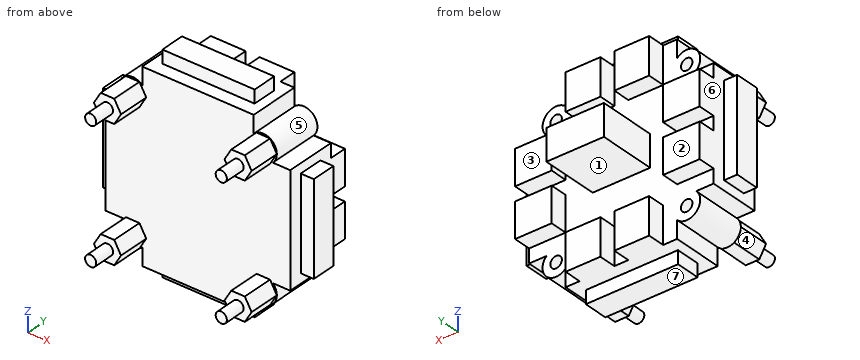
from build123d import *

# Parameters (mm, degrees)
SKETCH_1_R        = 3.889087297
SKETCH_1_R_2      = 1.65
EXTRUDE_2_DEPTH   = 7.25
EXTRUDE_2_2_DEPTH = 7.25
EXTRUDE_2_3_DEPTH = 7.25
EXTRUDE_2_4_DEPTH = 7.25
SKETCH_2_W        = 32
SKETCH_2_H        = 53
SKETCH_2_W_2      = 53
SKETCH_2_H_2      = 32
EXTRUDE_3_DEPTH   = 7.25
SKETCH_3_W        = 26.5
SKETCH_3_H        = 60.5
SKETCH_3_W_2      = 60.5
SKETCH_3_H_2      = 26.5
EXTRUDE_4_DEPTH   = 3.5
SKETCH_4_W        = 16.5
SKETCH_4_H        = 9
EXTRUDE_5_DEPTH   = 16.5
SKETCH_5_W        = 10.5
SKETCH_5_H        = 10
SKETCH_5_W_2      = 10
SKETCH_5_H_2      = 10.5
EXTRUDE_6_DEPTH   = 5
EXTRUDE_7_DEPTH   = 9
SKETCH_7_R        = 1.6
EXTRUDE_8_DEPTH   = 6


with BuildPart() as part:
    # Sketch 1 → Extrude 2 (new, symmetric)
    with BuildSketch(Plane(origin=(0, 0, 0), x_dir=(1, 0, 0), z_dir=(0, 1, 0))):
        with Locations(Location((-18.75, 18.75, 0), (0, 0, 90))):
            Circle(SKETCH_1_R)
        with Locations(Location((-18.75, 18.75, 0), (0, 0, 90))):
            Circle(SKETCH_1_R_2, mode=Mode.SUBTRACT)
    extrude(amount=EXTRUDE_2_DEPTH, both=True)



with BuildPart() as body_2:
    # Sketch 1 → Extrude 2 2 (new, symmetric)
    with BuildSketch(Plane(origin=(0, 0, 0), x_dir=(1, 0, 0), z_dir=(0, 1, 0))):
        with Locations(Location((18.75, 18.75, 0), (0, 0, 90))):
            Circle(SKETCH_1_R)
        with Locations(Location((18.75, 18.75, 0), (0, 0, 90))):
            Circle(SKETCH_1_R_2, mode=Mode.SUBTRACT)
    extrude(amount=EXTRUDE_2_2_DEPTH, both=True)


with BuildPart() as body_3:
    # Sketch 1 → Extrude 2 3 (new, symmetric)
    with BuildSketch(Plane(origin=(0, 0, 0), x_dir=(1, 0, 0), z_dir=(0, 1, 0))):
        with Locations(Location((18.75, -18.75, 0), (0, 0, 90))):
            Circle(SKETCH_1_R)
        with Locations(Location((18.75, -18.75, 0), (0, 0, 90))):
            Circle(SKETCH_1_R_2, mode=Mode.SUBTRACT)
    extrude(amount=EXTRUDE_2_3_DEPTH, both=True)


with BuildPart() as body_4:
    # Sketch 1 → Extrude 2 4 (new, symmetric)
    with BuildSketch(Plane(origin=(0, 0, 0), x_dir=(1, 0, 0), z_dir=(0, 1, 0))):
        with Locations(Location((-18.75, -18.75, 0), (0, 0, 90))):
            Circle(SKETCH_1_R)
        with Locations(Location((-18.75, -18.75, 0), (0, 0, 90))):
            Circle(SKETCH_1_R_2, mode=Mode.SUBTRACT)
    extrude(amount=EXTRUDE_2_4_DEPTH, both=True)


with BuildPart() as part_1:
    add(part.part)

    add(body_2.part)  # Extrude 3 merges body 2

    add(body_3.part)  # Extrude 3 merges body 3

    add(body_4.part)  # Extrude 3 merges body 4
    # Sketch 2 → Extrude 3 (add, symmetric)
    with BuildSketch(Plane(origin=(0, 0, 0), x_dir=(1, 0, 0), z_dir=(0, 1, 0))):
        Rectangle(SKETCH_2_W, SKETCH_2_H)
        Rectangle(SKETCH_2_W_2, SKETCH_2_H_2)
    extrude(amount=EXTRUDE_3_DEPTH, both=True)

    # Sketch 3 → Extrude 4 (add, symmetric)
    with BuildSketch(Plane(origin=(0, 0, 0), x_dir=(1, 0, 0), z_dir=(0, 1, 0))):
        Rectangle(SKETCH_3_W, SKETCH_3_H)
        Rectangle(SKETCH_3_W_2, SKETCH_3_H_2)
    extrude(amount=EXTRUDE_4_DEPTH, both=True)

    # Sketch 4 → Extrude 5 (add)
    with BuildSketch(Plane(origin=(0, 7.25, 0), x_dir=(1, 0, 0), z_dir=(0, 1, 0))):
        Rectangle(SKETCH_4_W, SKETCH_4_H)
    extrude(amount=EXTRUDE_5_DEPTH)

    # Sketch 5 → Extrude 6 (add)
    with BuildSketch(Plane(origin=(0, 7.25, 0), x_dir=(1, 0, 0), z_dir=(0, 1, 0))):
        with Locations((-21.25, 7)):
            Rectangle(SKETCH_5_W, SKETCH_5_H)
        with Locations((-21.25, -7)):
            Rectangle(SKETCH_5_W, SKETCH_5_H)
        with Locations((7, 21.25)):
            Rectangle(SKETCH_5_W_2, SKETCH_5_H_2)
        with Locations((-7, 21.25)):
            Rectangle(SKETCH_5_W_2, SKETCH_5_H_2)
        with Locations((21.25, -7)):
            Rectangle(SKETCH_5_W, SKETCH_5_H)
        with Locations((21.25, 7)):
            Rectangle(SKETCH_5_W, SKETCH_5_H)
        with Locations((-7, -21.25)):
            Rectangle(SKETCH_5_W_2, SKETCH_5_H_2)
        with Locations((7, -21.25)):
            Rectangle(SKETCH_5_W_2, SKETCH_5_H_2)
    extrude(amount=EXTRUDE_6_DEPTH)

    # Sketch 6 → Extrude 7 (add)
    with BuildSketch(Plane.XZ.offset(7.25)):
        Polygon((-14.860912703, 18.75), (-16.805456352, 22.118048396), (-20.694543648, 22.118048396), (-22.639087297, 18.75), (-20.694543648, 15.381951604), (-16.805456352, 15.381951604), align=None)
        Polygon((22.639087297, 18.75), (20.694543648, 22.118048396), (16.805456352, 22.118048396), (14.860912703, 18.75), (16.805456352, 15.381951604), (20.694543648, 15.381951604), align=None)
        Polygon((22.639087297, -18.75), (20.694543648, -15.381951604), (16.805456352, -15.381951604), (14.860912703, -18.75), (16.805456352, -22.118048396), (20.694543648, -22.118048396), align=None)
        Polygon((-14.860912703, -18.75), (-16.805456352, -15.381951604), (-20.694543648, -15.381951604), (-22.639087297, -18.75), (-20.694543648, -22.118048396), (-16.805456352, -22.118048396), align=None)
    extrude(amount=EXTRUDE_7_DEPTH)

    # Sketch 7 → Extrude 8 (add)
    with BuildSketch(Plane.XZ.offset(16.25)):
        with Locations(Location((-18.75, 18.75, 0), (0, 0, 270))):
            Circle(SKETCH_7_R)
        with Locations(Location((18.75, 18.75, 0), (0, 0, 270))):
            Circle(SKETCH_7_R)
        with Locations(Location((18.75, -18.75, 0), (0, 0, 270))):
            Circle(SKETCH_7_R)
        with Locations(Location((-18.75, -18.75, 0), (0, 0, 270))):
            Circle(SKETCH_7_R)
    extrude(amount=EXTRUDE_8_DEPTH)


solid = part_1.part
Work out the finished part from the listing and answer in its coordinate system (mm). Face numbers are marked on the shaded views. A direction names the side the tool comes from. Give positions to 0.01 mm unless a question says otherwise; leave off trailing zeros. Write each loop counter-clockwise with the first axis right and the second up, starting at its lowest first coordinate (ties: lowest second). Pieces come first, ordered by that corner, then holes.
Q1. The part is cut by section A-A on y = -11.5. Give the vertices of the cut face in (x, z), and give its area (3 significant figures).
Answer:
outline: (-22.64, -18.75) - (-20.69, -22.12) - (-16.81, -22.12) - (-14.86, -18.75) - (-16.81, -15.38) - (-20.69, -15.38) - close; (-22.64, 18.75) - (-20.69, 15.38) - (-16.81, 15.38) - (-14.86, 18.75) - (-16.81, 22.12) - (-20.69, 22.12) - close; (14.86, -18.75) - (16.81, -22.12) - (20.69, -22.12) - (22.64, -18.75) - (20.69, -15.38) - (16.81, -15.38) - close; (14.86, 18.75) - (16.81, 15.38) - (20.69, 15.38) - (22.64, 18.75) - (20.69, 22.12) - (16.81, 22.12) - close
area: 157 mm2
Q2. The part is cut by section B-B on x = 0. Give the vertices of the cut face in (y, z).
Answer:
outline: (-7.25, -26.5) - (-3.5, -26.5) - (-3.5, -30.25) - (3.5, -30.25) - (3.5, -26.5) - (7.25, -26.5) - (7.25, -4.5) - (23.75, -4.5) - (23.75, 4.5) - (7.25, 4.5) - (7.25, 26.5) - (3.5, 26.5) - (3.5, 30.25) - (-3.5, 30.25) - (-3.5, 26.5) - (-7.25, 26.5) - close
Q3. A tool of negligible diameter and unlimited length cuts with its end or side. For the marked faces 1, 2, 3 and 4, from which of +Z, -Z, +X, -X, +Y, -Y can it reach the whole face along a straight path? Write none if from no direction.
Answer:
face 1: +Y
face 2: +Z, -Z, -X, +Y
face 3: +Z, -Z, +X, +Y
face 4: -Z, -X, -Y
Q4. The part is cut by section D-D on y = 8.5. State how many separate pieces and enclosed holes the cut face has, and give its area (4 significant figures).
Answer:
separate pieces: 9
enclosed holes: 0
area: 988.5 mm2
Q5. For a pull along Z with two mould halves and no side action, classify the marked faces 5, 6 and 7 as released by +Z, released by -Z, zero draft, split by the parting line, or undercut.
Answer:
face 5: undercut
face 6: zero draft
face 7: released by -Z
Q6. Given pin 1 (2.5 mm diameter, centred on x = 5.5, y = 9, fed in from +Z); pin 2 (2 mm diameter, centred on x = 5, z = 23.5, fed in from -Y); pin 3 (4.5 mm diameter, centred on x = -18.5, y = -14, fed in from -Z), each flat-ended and moving along its own axis, determine where each tip first touches the part or whether it passes through.
Answer:
pin 1: stops at z = 26.5
pin 2: stops at y = -7.25
pin 3: stops at z = -22.12
Q7. Straight lines are drawn through the part: L1, parallel to Z at x = 18.75, y = -2.25; L2, parallel to Z at x = -18, y = 4. For each, find the intervals that lie inside material, in ascending order.
Answer:
L1: z = -22.64 to -20.4, -17.1 to 17.1, 20.4 to 22.64
L2: z = -22.57 to -20.22, -17.28 to 17.28, 20.22 to 22.57
Q8. The part is cut by section C-C on y = 17. Give the vertices of the cut face in (x, z), and give its area (4 significant figures).
Answer:
outline: (-8.25, -4.5) - (8.25, -4.5) - (8.25, 4.5) - (-8.25, 4.5) - close
area: 148.5 mm2
